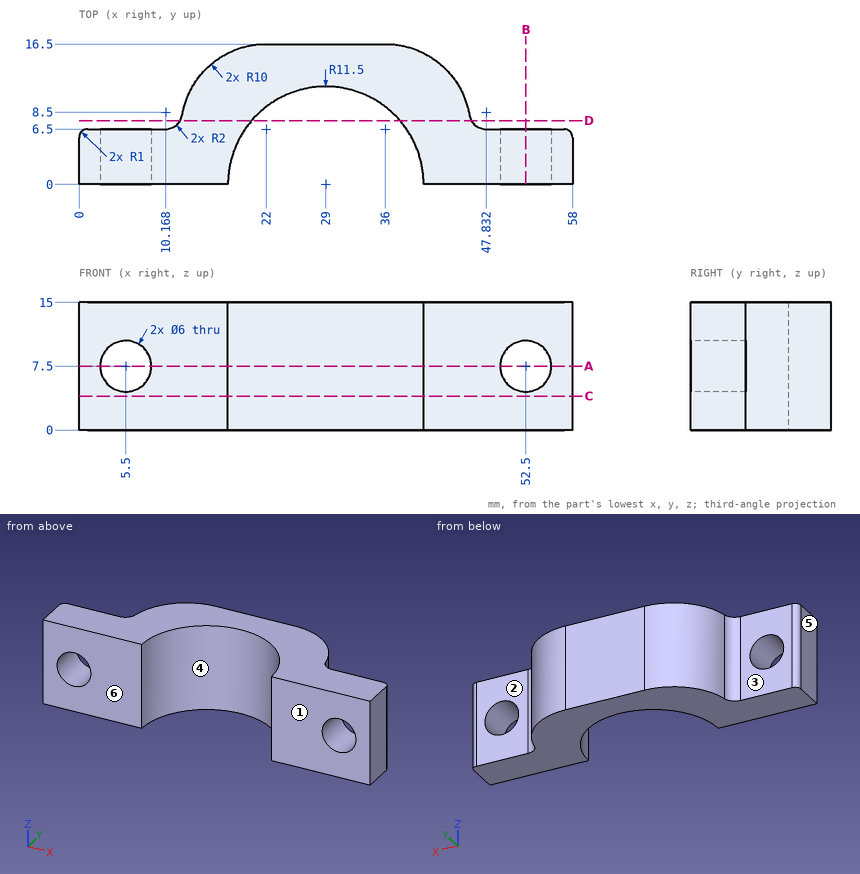
For this review, use the dimensioned drawing (mm, ordinates from the lowest corner) and the shaded views. A direction names the side the tool comes from. Coordinates: 2 decimals unless noted, no trailing zeros. Loops run counter-clockwise (first coordinate to the right, second up) from the corner with the lowest first, then second, coordinate; pieces in that order, holes last. Notation, with made-up numbers: M 18,-13 L 72,-13 A19 cw 72,-8 Z; hole C 77,47 d7. An arc over 180 degrees is marked long. Answer as CSV lines item,"result".
Item 1: The part is to be moulded in two halves that separate along X. For the marked faces 4, 5 and 6, say which applies: pulls with the +X half, pulls with the -X half, needs draft (parallel to the pull), parting line crosses it, or undercut.
Answer list:
face 4,"undercut"
face 5,"pulls with the -X half"
face 6,"needs draft"
Item 2: Add section B-B on x = 52.5. State the section outline as (y, z) points, plus the area to 3 significant figures.
Answer list:
outline,"M 0,0 L 6.5,0 L 6.5,4.5 L 0,4.5 Z; M 0,10.5 L 6.5,10.5 L 6.5,15 L 0,15 Z"
area,"58.5 mm²"
Item 3: Add section D-D on y = 7.5. State the section outline as (x, z) points, plus the area to 3 significant figures.
Answer list:
outline,"M 11.9,0 L 20.28,0 L 20.28,15 L 11.9,15 Z; M 37.72,0 L 46.1,0 L 46.1,15 L 37.72,15 Z"
area,"251 mm²"
Item 4: For probe 1 along Z at (x, y) = (5.5, 1.5); probe 2 along X at (y, z) = (2.5, 9.5) (1 decimal); probe 3 along X at (y, z) = (1.25, 10), list the stretches that pass through material, from the lowest coordinate up.
Answer list:
probe 1,"0 to 4.5, 10.5 to 15"
probe 2,"0 to 3.3, 7.7 to 17.8, 40.2 to 50.3, 54.7 to 58"
probe 3,"0 to 3.84, 7.16 to 17.57, 40.43 to 50.84, 54.16 to 58"
Item 5: For P1, Ø8, axis at x = 43, z = 4, coming from the +Y side; P2, Ø8, axis at x = 13.5, z = 7, coming from the +Y side; P3, Ø5.5, axis at x = 5.5, z = 7.5, coming from the +Y side; P4, Ø4, axis at y = 10, z = 10.5, coming from the -X side, all flat-tipped, find the tip position at first contact; note any pin that passes through.
Answer list:
P1,"y = 16.04"
P2,"y = 15.43"
P3,"through"
P4,"x = 12.1"
Item 6: Add section A-A on z = 7.5. State the section outline as (x, y) points, plus the area to 3 significant figures.
Answer list:
outline,"M 0,0 L 2.5,0 L 2.5,6.5 L 1,6.5 A1 ccw 0,5.5 Z; M 8.5,0 L 17.5,0 A11.5 cw 40.5,0 L 49.5,0 L 49.5,6.5 L 47.83,6.5 A2 cw 45.86,8.17 A10 ccw 36,16.5 L 22,16.5 A10 ccw 12.14,8.17 A2 cw 10.17,6.5 L 8.5,6.5 Z; M 55.5,0 L 58,0 L 58,5.5 A1 ccw 57,6.5 L 55.5,6.5 Z"
area,"389 mm²"
Item 7: Add section C-C on z = 4. State the section outline as (x, y) points, plus the area to 3 significant figures.
Answer list:
outline,"M 0,0 L 17.5,0 A11.5 cw 40.5,0 L 58,0 L 58,5.5 A1 ccw 57,6.5 L 47.83,6.5 A2 cw 45.86,8.17 A10 ccw 36,16.5 L 22,16.5 A10 ccw 12.14,8.17 A2 cw 10.17,6.5 L 1,6.5 A1 ccw 0,5.5 Z"
area,"467 mm²"
Item 8: Machinability: for the marked faces 1, 2 and 3, which of the approach directions +Z, -Z, +X, -X, +Y, -Y give a long, thin tool a straight path to every point of the face, cutting with its end or side? Answer none if there is none.
Answer list:
face 1,"+Z, -Z, +X, -X, -Y"
face 2,"+Z, -Z, +X, +Y"
face 3,"+Z, -Z, -X, +Y"
